Part model, mm, in its own coordinate system. Face numbers are marked on the shaded views. A direction names the side the tool comes from. Coordinates: 2 decimals unless noted, no trailing zeros. Loops run counter-clockwise (first coordinate to the right, second up) from the corner with the lowest first, then second, coordinate; pieces in that order, holes last. Notation, with made-up numbers: M 10.25,37.25 L 16.25,37.25 A28 ccw 16.25,56.25 Z; hole C -31,-14.5 d3. An arc over 180 degrees is marked long. Use a Markdown table: item, result. Add a question column.
1) Pin check, flat tips, straight feed: pin 1 Ø0.6 at (x, y) = (8.5, 26) entering from -Z; pin 2 Ø1.5 at (x, y) = (4, 10) entering from +Z; pin 3 Ø3 at (x, y) = (0, 4.8) entering from +Z. Stop position of each tip, or through.
2) Band-saw the part on C-C (z = 12.75). List the corners of the cut face in (x, y).
3) Band-saw the part on D-D (y = 18.5). List the corners of the cut face in (x, z).
4) Band-saw the part on A-A (x = 0). List the corners of the cut face in (y, z).
5) Band-saw the part on B-B (y = 4.8). List the corners of the cut face in (x, z), plus the area to 3 significant figures.
6) Tool access for the marked faces 1 and 2: list every direction of +Z, -Z, +X, -X, +Y, -Y with a clear straight run to the whole face (end or side of a thin tool).
7) Wall check: probe 1 along X at (y, z) = (12.8, 1.1); probe 2 along Y at (x, z) = (0, 0.4); probe 3 along Y at (x, z) = (0, 1.1). Give the ranges that are in metal, low to high. Write a range as from..to.
8) Pull direction Y, two halves, no side cores. Call the marked faces 3, 4 and 5: released by +Y, released by -Y, zero draft, split by the parting line, or undercut.
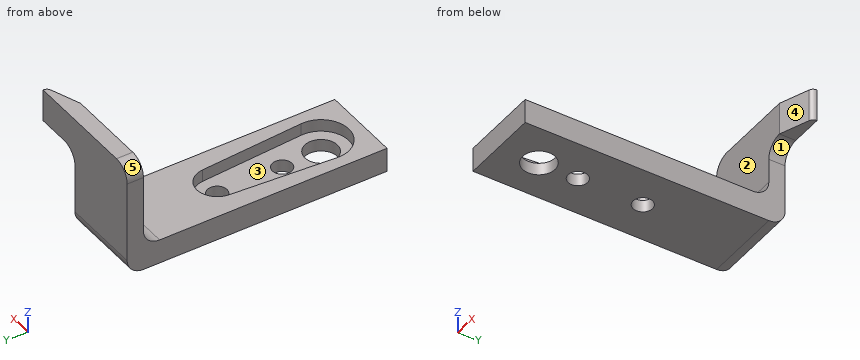
from build123d import *

# Parameters (mm, degrees)
F0_W      = 9.8
F0_H      = 32
F0_R      = 2
F0_R_2    = 1.2
F1_DEPTH  = 3
F3_DEPTH  = 1.5
F4_W      = 9.8
F4_H      = 2
F5_DEPTH  = 11
F6_W      = 2
F6_H      = 4
F7_DEPTH  = 6
F8_R      = 2
F10_DEPTH = 4


with BuildPart() as f1:
    # F0 (on Top) → F1 (new body)
    with BuildSketch(Plane.XY):
        with Locations((0, 11.1)):
            Rectangle(F0_W, F0_H)
        Circle(F0_R, mode=Mode.SUBTRACT)
        with Locations((0, 4.8)):
            Circle(F0_R_2, mode=Mode.SUBTRACT)
        with Locations((0, 12.8)):
            Circle(F0_R_2, mode=Mode.SUBTRACT)
    extrude(amount=F1_DEPTH)

    # F2 (on face) → F3 (cut)
    with BuildSketch(Plane.XY.offset(3)):
        with BuildLine():
            Line((-2.493813, 12.975781), (-3.391585, 0.239062))
            ThreePointArc((-3.391585, 0.239062), (0, -3.4), (3.391585, 0.239062))
            Line((3.391585, 0.239062), (2.493813, 12.975781))
            ThreePointArc((2.493813, 12.975781), (0, 15.3), (-2.493813, 12.975781))
        make_face()
    extrude(amount=-F3_DEPTH, mode=Mode.SUBTRACT)

    # F4 (on face) → F5 (join)
    with BuildSketch(Plane.XY.offset(3)):
        with Locations((0, 26.1)):
            Rectangle(F4_W, F4_H)
    extrude(amount=F5_DEPTH)

    # F6 (on face) → F7 (join)
    with BuildSketch(Plane.YZ.offset(4.9)):
        with Locations((26.1, 12)):
            Rectangle(F6_W, F6_H)
    extrude(amount=F7_DEPTH)

    # F8
    f8_edges = [f1.edges().sort_by_distance(p)[0] for p in [
        (4.9, 26.1, 10),
        (-4.9, 26.1, 14),
        (0, 25.1, 3),
        (0, 27.1, 0),
    ]]
    fillet(f8_edges, radius=F8_R)

    # F9 (on face) → F10 (cut, through all)
    with BuildSketch(Plane(origin=(0, 0, 10), x_dir=(1, 0, 0), z_dir=(0, 0, -1))):
        with BuildLine():
            Line((10.9, -25.1), (6.9, -25.1))
            Line((6.9, -25.1), (10.431835, -26.424438))
            ThreePointArc((10.431835, -26.424438), (10.771519, -26.689037), (10.9, -27.1))
            Line((10.9, -27.1), (10.9, -26.6))
            Line((10.9, -26.6), (10.9, -25.1))
        make_face()
    extrude(amount=-F10_DEPTH, mode=Mode.SUBTRACT)


solid = f1.part
Entries:
| question | item | result |
|---|---|---|
| 1 | pin 1 | z = 10 |
| 1 | pin 2 | z = 3 |
| 1 | pin 3 | z = 1.5 |
| 2 | outline | M -4.75,25.1 L 6.9,25.1 L 10.43,26.42 A0.72 ccw 10.9,27.1 L -4.75,27.1 Z |
| 3 | outline | M -4.9,0 L 4.9,0 L 4.9,3 L -4.9,3 Z |
| 4 | outline | M -4.9,0 L -2,0 L -2,1.5 L -3.4,1.5 L -3.4,3 L -4.9,3 Z; M 2,0 L 3.6,0 L 3.6,1.5 L 2,1.5 Z; M 6,0 L 11.6,0 L 11.6,1.5 L 6,1.5 Z; M 14,0 L 25.1,0 A2 ccw 27.1,2 L 27.1,14 L 25.1,14 L 25.1,5 A2 cw 23.1,3 L 15.3,3 L 15.3,1.5 L 14,1.5 Z |
| 5 | outline | M -4.9,0 L -1.2,0 L -1.2,1.5 L -3.07,1.5 L -3.07,3 L -4.9,3 Z; M 1.2,0 L 4.9,0 L 4.9,3 L 3.07,3 L 3.07,1.5 L 1.2,1.5 Z |
| 5 | area | 16.6 mm2 |
| 6 | face 1 | -Z, +X, +Y, -Y |
| 6 | face 2 | +Z, +X, -X, -Y |
| 7 | probe 1 | -4.9..-1.2, 1.2..4.9 |
| 7 | probe 2 | -4.9..-2, 2..3.6, 6..11.6, 14..26.3 |
| 7 | probe 3 | -4.9..-2, 2..3.6, 6..11.6, 14..26.89 |
| 8 | face 3 | undercut |
| 8 | face 4 | released by -Y |
| 8 | face 5 | zero draft |
